Geometry: final body of the model. Coordinates: model frame, mm. Face numbers are marked on the shaded views. A direction names the side the tool comes from. Coordinates: 2 decimals unless noted, no trailing zeros. Write each loop counter-clockwise with the first axis right and the second up, starting at its lowest first coordinate (ties: lowest second). Pieces come first, ordered by that corner, then holes. Notation, with made-up numbers: (-27.5, -22.5) -> (9.5, -22.5) arc R26 ccw to (9.5, 16.5) -> close; hole circle Ø1 at (17.25, -24). An arc over 180 degrees is marked (long way). One line per item, written item: value. Start each with the question number.
from build123d import *

# Parameters (mm, degrees)
F0_W     = 51.0519817472
F0_H     = 50.4617840052
F1_DEPTH = 67.3618763685
F2_R     = 12.5571720672
F3_DEPTH = 39.3777489662
F4_W     = 44.3657840052
F4_H     = 61.2658763685
F5_DEPTH = 25.4


with BuildPart() as f1:
    # F0 (on Top) → F1 (new body)
    with BuildSketch(Plane.XY):
        with Locations((-0.7996745408, 10.5232298374)):
            Rectangle(F0_W, F0_H)
    extrude(amount=F1_DEPTH)

    # F2 (on face) → F3 (join)
    with BuildSketch(Plane.XZ.offset(14.7076621652)):
        with Locations((7.6489895582, 49.6433377266)):
            Circle(F2_R)
    extrude(amount=F3_DEPTH)

    # F4 (on face) → F5 (join)
    with BuildSketch(Plane(origin=(-26.3256654143, 0, 0), x_dir=(0, -1, 0), z_dir=(-1, 0, 0))):
        with Locations((-10.5232298374, 33.6809381843)):
            Rectangle(F4_W, F4_H)
    extrude(amount=F5_DEPTH)


solid = f1.part
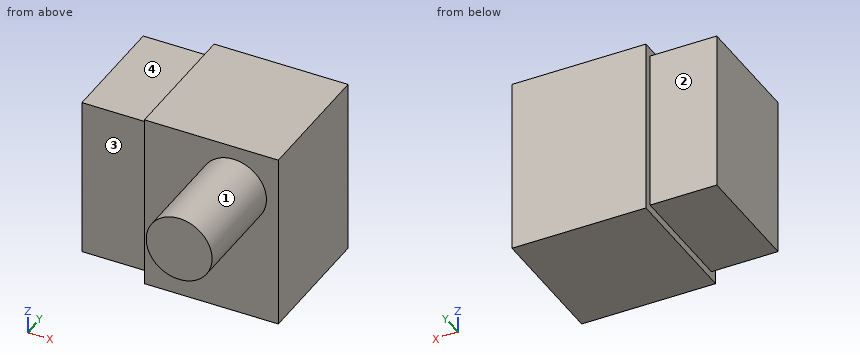
Q1. Cut plane C-C on x = -36. Output: boundary loops of the cut face in (y, z).
Q2. Cut plane D-D on z = 54.5. Output: boundary loops of the cut face in (x, y).
Q3. Cut plane B-B on y = 25.5. Output: boundary loops of the cut face in (x, z), and give its area (3 significant figures).
Q4. Access query for the marked faces 1, 2, 3 and 4. Directions: +Z, -Z, +X, -X, +Y, -Y. A direction counts if a zero-diameter tool reaches every point of the face in a straight line with its end or side. Return the directions, or none.
Q5. First-contact query: P1, Ø7.5, axis at x = -39.5, z = 36.5, coming from the +Y side; P2, Ø20.5, axis at x = -40, z = 36.5, coming from the -Y side; P3, Ø12, axis at x = -5, z = 57, coming from the -Y side; P4, Ø12.5, axis at x = -36.5, y = 12, coming from the -Z side. Flat tips, straight axial feed; report the tip coordinate or a pass-through.
Q6. Line query: L1, parallel to Z at x = -39, y = 29.5; L2, parallel to Y at x = -38, z = 19.5; L3, parallel to Y at x = 3, z = 8. Output: solid intervals per line, ascending. Write a range as from..to.
Q7. Cut plane A-A on z = 5.5. Output: boundary loops of the cut face in (x, y), and give its area (3 significant figures).
Solution:
1. outline: (-11.66, 3.05) -> (32.71, 3.05) -> (32.71, 64.31) -> (-11.66, 64.31) -> close
2. outline: (-51.73, -11.66) -> (-26.33, -11.66) -> (-26.33, -14.71) -> (-3.93, -14.71) -> (-3.93, -54.09) -> (19.23, -54.09) -> (19.23, -14.71) -> (24.73, -14.71) -> (24.73, 35.75) -> (-26.33, 35.75) -> (-26.33, 32.71) -> (-51.73, 32.71) -> close
3. outline: (-51.73, 3.05) -> (-26.33, 3.05) -> (-26.33, 0) -> (24.73, 0) -> (24.73, 67.36) -> (-26.33, 67.36) -> (-26.33, 64.31) -> (-51.73, 64.31) -> close
3. area: 5,000 mm²
4. face 1: -Y
4. face 2: +Z, -Z, -X, +Y
4. face 3: +Z, -Z, -X, -Y
4. face 4: +Z, -X, +Y, -Y
5. P1: y = 32.71
5. P2: y = -11.66
5. P3: y = -54.09
5. P4: z = 3.05
6. L1: 3.05..64.31
6. L2: -11.66..32.71
6. L3: -14.71..35.75
7. outline: (-51.73, -11.66) -> (-26.33, -11.66) -> (-26.33, -14.71) -> (24.73, -14.71) -> (24.73, 35.75) -> (-26.33, 35.75) -> (-26.33, 32.71) -> (-51.73, 32.71) -> close
7. area: 3,700 mm²
